CAD build for the part. Positions are in the model's coordinates, mm. Face numbers are marked on the shaded views. A direction names the side the tool comes from. Round coordinates to 2 decimals unless told otherwise and drop trailing zeros. Loops run counter-clockwise (first coordinate to the right, second up) from the corner with the lowest first, then second, coordinate; pieces in that order, holes last. Notation, with made-up numbers: M 75.25,76.5 L 107.25,76.5 A26 cw 107.25,112.5 Z; hole C 17,-20 d6. An arc over 180 degrees is marked long. Use one line per item in the form item = value.
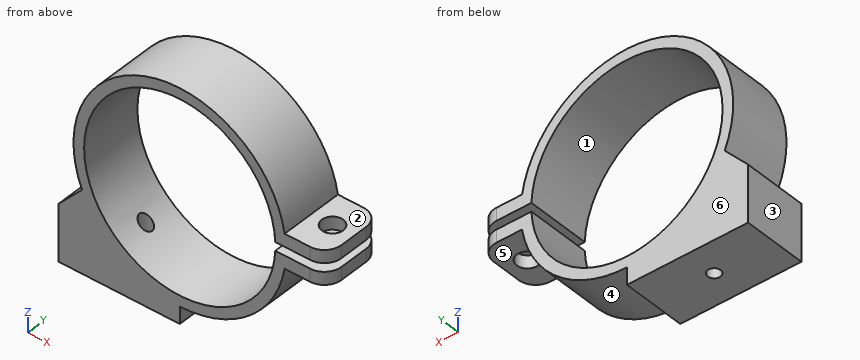
from build123d import *

# Parameters (mm, degrees)
SALIENTE_EXTRUIR1_DEPTH = 15
CROQUIS2_R              = 1.5
CORTAR_EXTRUIR1_DEPTH   = 17
CROQUIS3_R              = 2.5
CORTAR_EXTRUIR2_DEPTH   = 17
REDONDEO1_R             = 4


with BuildPart() as part:
    # Croquis1 → Saliente-Extruir1 (new body)
    with BuildSketch(Plane(origin=(0, 0, 0), x_dir=(1, 0, 0), z_dir=(0, 1, 0))):
        with BuildLine():
            Line((0, 25), (0, 29))
            Line((0, 29), (-28.5, 29))
            Line((-28.5, 29), (-28.5, 15.712290503))
            Line((-28.5, 15.712290503), (-22.998889471, 9.800565448))
            ThreePointArc((-22.998889471, 9.800565448), (-6.951164798, -24.014189721), (24.677925359, -4))
            Line((24.677925359, -4), (34.677925359, -4))
            Line((34.677925359, -4), (34.677925359, -1))
            Line((34.677925359, -1), (22.477766793, -1))
            ThreePointArc((22.477766793, -1), (-22.5, 0), (22.477766793, 1))
            Line((22.477766793, 1), (34.677925359, 1))
            Line((34.677925359, 1), (34.677925359, 4))
            Line((34.677925359, 4), (24.677925359, 4))
            ThreePointArc((24.677925359, 4), (16.201851746, 19.039432765), (0, 25))
        make_face()
    extrude(amount=SALIENTE_EXTRUIR1_DEPTH)

    # Croquis2 → Cortar-Extruir1 (cut)
    with BuildSketch(Plane(origin=(0, 0, -29), x_dir=(-1, 0, 0), z_dir=(0, 0, -1))):
        with Locations((14.25, 7.5)):
            Circle(CROQUIS2_R)
    extrude(amount=-CORTAR_EXTRUIR1_DEPTH, mode=Mode.SUBTRACT)

    # Croquis3 → Cortar-Extruir2 (cut)
    with BuildSketch(Plane(origin=(0, 0, -4), x_dir=(-1, 0, 0), z_dir=(0, 0, -1))):
        with Locations((-29.677925359, 7.5)):
            Circle(CROQUIS3_R)
    extrude(amount=-CORTAR_EXTRUIR2_DEPTH, mode=Mode.SUBTRACT)

    # Redondeo1
    redondeo1_edges = [part.edges().sort_by_distance(p)[0] for p in [
        (34.677925359, 0, -2.5),
        (34.677925359, 0, 2.5),
        (34.677925359, 15, 2.5),
        (34.677925359, 15, -2.5),
    ]]
    fillet(redondeo1_edges, radius=REDONDEO1_R)


solid = part.part
1. Probe line 1 along Y through (x, z) = (-14.25, -23.75); line 2 along Z through (x, y) = (25.5, 1); line 3 along Z through (x, y) = (-9, 6.25). List the from-to ranges inside material, lowest first. Write a range as from..to.
Completed:
line_1 = 0..6, 9..15
line_2 = -4..-1, 1..4
line_3 = -29..-20.62, 20.62..23.32
2. Cut at D-D on z = 0. Write the cut outline in (x, y).
Completed:
outline = M -25,0 L -22.5,0 L -22.5,15 L -25,15 Z
3. Pull direction Z, two halves, no side cores. Call the marked faces 1, 2, 3 and 4: +Z half, -Z half, draft (parallel to the pull), parting line (faces both ways), or undercut.
Completed:
face_1 = undercut
face_2 = +Z half
face_3 = draft
face_4 = -Z half
4. Drop flat-ended pins along their axis: P1, Ø6, axis at y = 4, z = -1.5, coming from the -X side; P2, Ø4, axis at x = 14.5, y = 9, coming from the -Z side; P3, Ø3, axis at y = 13, z = 9.5, coming from the -X side; P4, Ø3.5, axis at x = -14.25, y = 7.5, coming from the -Z side. Give the stop position or say it passes through.
Completed:
P1 = -25
P2 = -21.65
P3 = -23.69
P4 = -29
5. Cut at A-A on x = -14.25. Write the cut outline in (y, z).
Completed:
outline = M 0,-29 L 6,-29 L 6,-17.41 L 0,-17.41 Z; M 0,17.41 L 15,17.41 L 15,20.54 L 0,20.54 Z; M 9,-29 L 15,-29 L 15,-17.41 L 9,-17.41 Z
6. Cut at B-B on y = 7.5. Write the cut outline in (x, z).
Completed:
outline = M -28.5,-29 L -15.75,-29 L -15.75,-16.07 A22.5 cw long 22.48,1 L 27.18,1 L 27.18,4 L 24.68,4 A25 ccw long -23,-9.8 L -28.5,-15.71 Z; M -12.75,-29 L 0,-29 L 0,-25 A25 ccw 24.68,-4 L 27.18,-4 L 27.18,-1 L 22.48,-1 A22.5 cw -12.75,-18.54 Z; M 32.18,-4 L 34.68,-4 L 34.68,-1 L 32.18,-1 Z; M 32.18,1 L 34.68,1 L 34.68,4 L 32.18,4 Z
7. Tool access for the marked faces 5 and 6: list every direction of +Z, -Z, +X, -X, +Y, -Y with a clear straight run to the whole face (end or side of a thin tool).
Completed:
face_5 = -Z, +X, +Y, -Y
face_6 = +Z, -Z, +X, -X, +Y
8. Cut at C-C on z = -11. Write the cut outline in (x, y).
Completed:
outline = M -24.12,0 L -19.63,0 L -19.63,15 L -24.12,15 Z; M 19.63,0 L 22.45,0 L 22.45,15 L 19.63,15 Z
